from build123d import *

# Parameters (mm, degrees)
BOSS_EXTRUDE1_START     = -5
BOSS_EXTRUDE1_OUTLINE_R = 1.75
BOSS_EXTRUDE1_DEPTH     = 5
SKETCH3_W               = 25
SKETCH3_H               = 4
BOSS_EXTRUDE2_DEPTH     = 20
SKETCH4_R               = 1.75
CUT_EXTRUDE1_DEPTH      = 4
BOSS_EXTRUDE3_DEPTH     = 25
FILLET2_R               = 2


with BuildPart() as part:
    # Boss-Extrude1: read off the stored shape, not the designer's step
    # Boss-Extrude1 outline → Boss-Extrude1 (new body)
    with BuildSketch(Plane(origin=(5, 0, 0), x_dir=(0, 0, -1), z_dir=(1, 0, 0)).offset(BOSS_EXTRUDE1_START)):
        with BuildLine():
            Line((-6.17, -30), (6.17, -30))
            ThreePointArc((6.17, -30), (12.413752878, -27.413752878), (15, -21.17))
            Line((15, -21.17), (15, -13.83))
            Line((15, -13.83), (18.5, -13.83))
            Line((18.5, -13.83), (18.5, -3.83))
            Line((18.5, -3.83), (15, -3.83))
            Line((15, -3.83), (15, 6.17))
            Line((15, 6.17), (18.5, 6.17))
            Line((18.5, 6.17), (18.5, 16.17))
            Line((18.5, 16.17), (15, 16.17))
            Line((15, 16.17), (15, 21.17))
            ThreePointArc((15, 21.17), (12.413752878, 27.413752878), (6.17, 30))
            Line((6.17, 30), (-6.17, 30))
            ThreePointArc((-6.17, 30), (-12.413752878, 27.413752878), (-15, 21.17))
            Line((-15, 21.17), (-15, 16.17))
            Line((-15, 16.17), (-18.5, 16.17))
            Line((-18.5, 16.17), (-18.5, 6.17))
            Line((-18.5, 6.17), (-15, 6.17))
            Line((-15, 6.17), (-15, -3.83))
            Line((-15, -3.83), (-18.5, -3.83))
            Line((-18.5, -3.83), (-18.5, -13.83))
            Line((-18.5, -13.83), (-15, -13.83))
            Line((-15, -13.83), (-15, -21.17))
            ThreePointArc((-15, -21.17), (-12.413752878, -27.413752878), (-6.17, -30))
        make_face()
        with Locations((-4.875, -24.3)):
            Circle(BOSS_EXTRUDE1_OUTLINE_R, mode=Mode.SUBTRACT)
        with Locations((4.875, -24.3)):
            Circle(BOSS_EXTRUDE1_OUTLINE_R, mode=Mode.SUBTRACT)
        with Locations((-4.875, 24.3)):
            Circle(BOSS_EXTRUDE1_OUTLINE_R, mode=Mode.SUBTRACT)
        with Locations((4.875, 24.3)):
            Circle(BOSS_EXTRUDE1_OUTLINE_R, mode=Mode.SUBTRACT)
    extrude(amount=BOSS_EXTRUDE1_DEPTH)

    # Sketch3 → Boss-Extrude2 (add)
    with BuildSketch(Plane.ZY):
        with Locations((0, -13.83)):
            Rectangle(SKETCH3_W, SKETCH3_H)
    extrude(amount=BOSS_EXTRUDE2_DEPTH)

    # Sketch4 → Cut-Extrude1 (cut)
    with BuildSketch(Plane.XZ.offset(15.83)):
        with Locations(Location((-16.5, -8.8, 0), (0, 0, 270))):
            Circle(SKETCH4_R)
        with Locations(Location((-16.5, 8.8, 0), (0, 0, 90))):
            Circle(SKETCH4_R)
    extrude(amount=-CUT_EXTRUDE1_DEPTH, mode=Mode.SUBTRACT)

    # Sketch6 → Boss-Extrude3 (add)
    with BuildSketch(Plane.XY.offset(12.5)):
        Polygon((0, -11.83), (1.101299034, -11.83), (1.101299034, -6.83), (0, -6.83), (-5.038932071, -11.83), align=None)
        Polygon((-5.038932071, -15.83), (0, -15.83), (1.101299034, -15.83), (1.101299034, -20.83), (0, -20.83), align=None)
    extrude(amount=-BOSS_EXTRUDE3_DEPTH)

    # Fillet2
    fillet2_edges = [part.edges().sort_by_distance(p)[0] for p in [
        (0, -6.83, 0),
        (-5.038932071, -11.83, 0),
        (-5.038932071, -15.83, 0),
        (0, -20.83, 0),
    ]]
    fillet(fillet2_edges, radius=FILLET2_R)


solid = part.part
Verification items for the finished model (mm, model axes). A direction names the side the tool comes from. Round coordinates to 2 decimals unless told otherwise and drop trailing zeros. Loops run counter-clockwise (first coordinate to the right, second up) from the corner with the lowest first, then second, coordinate; pieces in that order, holes last. Notation, with made-up numbers: (-8.5, 53) - (26.5, 53) arc R30 cw to (26.5, 90) - close; hole circle Ø4 at (70, 20). An arc over 180 degrees is marked (long way). Use a Markdown table: item, result. Add a question column.
1. Thickness scan on probe 1 along X at (y, z) = (-14.8, 8.8); probe 2 along Z at (x, y) = (-17, -12); probe 3 along X at (y, z) = (14, -1.5). Record the ranges inside material, lowest first. Write a range as [from, to].
2. Release check for a two-part mould opening along Z. For faces 6 (the face through (2, 1, -15)), 7 (the face through (-14.765, -13.858, -8.572)), 8 (the face through (-5.091, -15.985, -0.175)), 9 (the face through (2.465, 26.035, 5.103)) record: released by +Z, released by -Z, zero draft, split by the parting line, or undercut.
3. Section check A-A, the plane x = -16.5. Record the boundary of the cut face in (y, z).
4. Section check D-D, the plane y = -24.3. Record the boundary of the cut face in (x, z) (3 decimals).
5. Gauge pin test, flat ends, axial feed: pin 1 (4 mm diameter, centred on x = -12.5, z = -0.5, fed in from -Y); pin 2 (4 mm diameter, centred on x = -7, z = 0, fed in from -Y); pin 3 (5 mm diameter, centred on y = -23.5, z = -4.5, fed in from -X). Record the tip position at first contact, or that the pin passes through.
6. Section check C-C, the plane z = 16. Record the boundary of the cut face in (x, y), plus the area to 3 significant figures.
7. Section check B-B, the plane y = -15. Record the boundary of the cut face in (x, z), plus the area to 3 significant figures.
8. Access from +Z, -Z, +X, -X, +Y, -Y to the whole of each face (thin tool, end or side, straight path). Record for faces 1 (the face through (2, 16.17, 17)), 2 (the face through (-5.111, -11.683, -0.175)), 3 (the face through (2, -18, -15)), 4 (the face through (2, 19, -15)), 5 (the face through (2, -30, 0)).
Checks:
| question | item | result |
|---|---|---|
| 1 | probe 1 | x = [-20, -18.25], [-14.75, 5] |
| 1 | probe 2 | z = [-12.5, -10.48], [-7.12, 7.12], [10.48, 12.5] |
| 1 | probe 3 | x = [0, 5] |
| 2 | face 6 | released by -Z |
| 2 | face 7 | undercut |
| 2 | face 8 | zero draft |
| 2 | face 9 | undercut |
| 3 | outline | (-15.83, -12.5) - (-11.83, -12.5) - (-11.83, -10.55) - (-15.83, -10.55) - close; (-15.83, -7.05) - (-11.83, -7.05) - (-11.83, 7.05) - (-15.83, 7.05) - close; (-15.83, 10.55) - (-11.83, 10.55) - (-11.83, 12.5) - (-15.83, 12.5) - close |
| 4 | outline | (0, -14.427) - (5, -14.427) - (5, -6.625) - (0, -6.625) - close; (0, -3.125) - (5, -3.125) - (5, 3.125) - (0, 3.125) - close; (0, 6.625) - (5, 6.625) - (5, 14.427) - (0, 14.427) - close |
| 5 | pin 1 | stops at y = -15.83 |
| 5 | pin 2 | stops at y = -16.03 |
| 5 | pin 3 | stops at x = -0.11 |
| 6 | outline | (0, -13.83) - (5, -13.83) - (5, -3.83) - (0, -3.83) - close; (0, 6.17) - (5, 6.17) - (5, 16.17) - (0, 16.17) - close |
| 6 | area | 100 mm^2 |
| 7 | outline | (-20, -12.5) - (0, -12.5) - (0, -15) - (5, -15) - (5, 15) - (0, 15) - (0, 12.5) - (-20, 12.5) - close; hole circle Ø3.5 at (-16.5, -8.8); hole circle Ø3.5 at (-16.5, 8.8) |
| 7 | area | 631 mm^2 |
| 8 | face 1 | +Z, +X, -X, +Y |
| 8 | face 2 | +Z, -Z, -X, +Y |
| 8 | face 3 | -Z, +X, -X, -Y |
| 8 | face 4 | -Z, +X, -X, +Y |
| 8 | face 5 | +Z, -Z, +X, -X, -Y |
